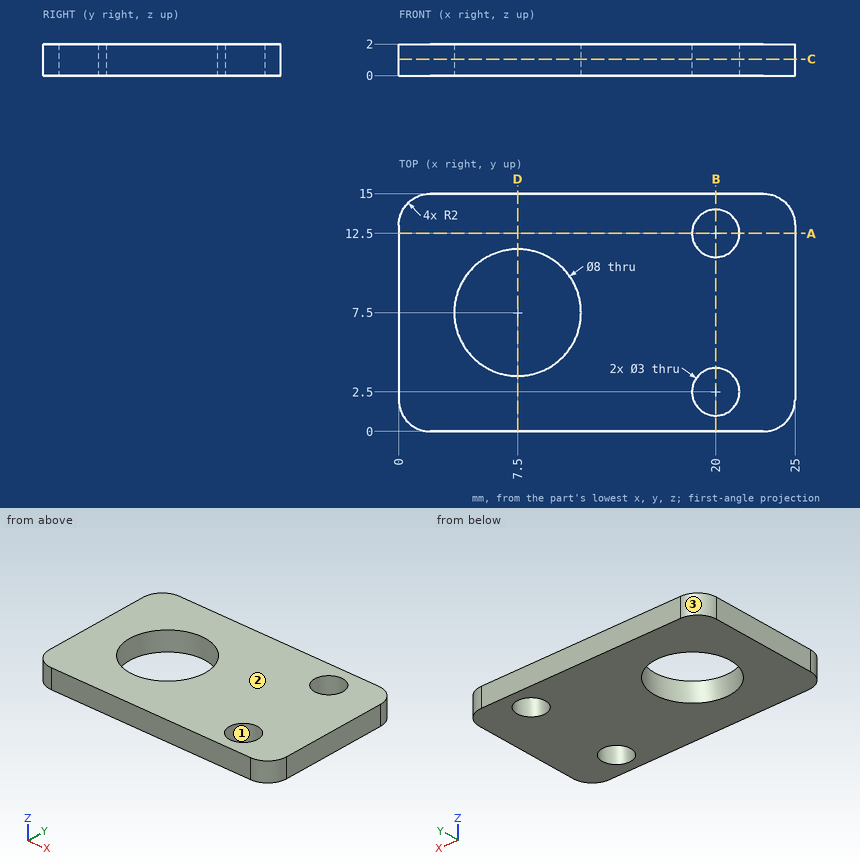
Geometry check sheet. Reference: drawing and pictorial views, mm from the part's lowest x, y, z. Give positions to 0.01 mm unless a question says otherwise; leave off trailing zeros. Write each loop counter-clockwise with the first axis right and the second up, starting at its lowest first coordinate (ties: lowest second). Pieces come first, ordered by that corner, then holes.
Item 1: Gauge pin test, flat end, axial feed: pin 1 (2.5 mm diameter, centred on x = 20, y = 12.5, fed in from +Z). Record the tip position at first contact, or that the pin passes through.
Item 2: Cross-section at B-B (x = 20). Enter the section's corners in (y, z).
Item 3: Scan lines: L1, parallel to Y at x = 20, z = 0.45; L2, parallel to Y at x = 7.5, z = 1.15; L3, parallel to Y at x = 19.25, z = 1.95. Record each from-to range of solid material in increasing order.
Item 4: Cross-section at D-D (x = 7.5). Enter the section's corners in (y, z).
Item 5: Draft check along Y on the marked faces 1, 2 and 3. Enter one of: released by +Y, released by -Y, zero draft, split by the parting line, or undercut.
Item 6: Cross-section at A-A (y = 12.5). Enter the section's corners in (x, z), and give its area (3 significant figures).
Item 7: Cross-section at C-C (z = 1.05). Enter the section's corners in (x, y), and give its area (3 significant figures).
Report:
1. pin 1: passes through
2. outline: (0, 0) - (1, 0) - (1, 2) - (0, 2) - close; (4, 0) - (11, 0) - (11, 2) - (4, 2) - close; (14, 0) - (15, 0) - (15, 2) - (14, 2) - close
3. L1: y = 0 to 1, 4 to 11, 14 to 15
3. L2: y = 0 to 3.5, 11.5 to 15
3. L3: y = 0 to 1.2, 3.8 to 11.2, 13.8 to 15
4. outline: (0, 0) - (3.5, 0) - (3.5, 2) - (0, 2) - close; (11.5, 0) - (15, 0) - (15, 2) - (11.5, 2) - close
5. face 1: undercut
5. face 2: zero draft
5. face 3: released by +Y
6. outline: (0, 0) - (18.5, 0) - (18.5, 2) - (0, 2) - close; (21.5, 0) - (25, 0) - (25, 2) - (21.5, 2) - close
6. area: 44.0 mm2
7. outline: (0, 2) arc R2 ccw to (2, 0) - (23, 0) arc R2 ccw to (25, 2) - (25, 13) arc R2 ccw to (23, 15) - (2, 15) arc R2 ccw to (0, 13) - close; hole circle Ø8 at (7.5, 7.5); hole circle Ø3 at (20, 2.5); hole circle Ø3 at (20, 12.5)
7. area: 307 mm2
